For this review, take the finished solid that the model builds, in its own axes (mm). Face numbers are marked on the shaded views. Round coordinates to 2 decimals unless told otherwise and drop trailing zeros. Order: outer loops, then holes, each group sorted by start corner. A loop starts at its lowest first (then second) coordinate and runs counter-clockwise, first axis right, second up. Notation, with made-up numbers: M 67.25,44 L 103.25,44 A34 cw 103.25,81 Z; hole C 32.25,26 d3. An arc over 180 degrees is marked long. Use a Markdown table: item, result.
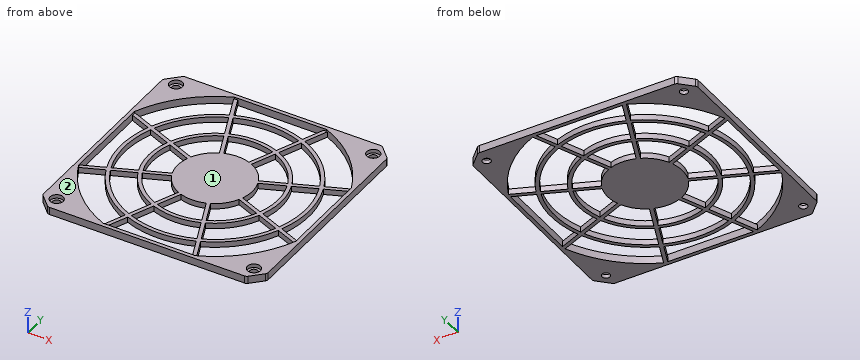
from build123d import *

# Parameters (mm, degrees)
SKETCH1_W           = 120
SKETCH1_H           = 120
SKETCH1_R           = 2.15
BOSS_EXTRUDE1_DEPTH = 4
CHAMFER1_SIZE       = 7
SKETCH2_R           = 20
BOSS_EXTRUDE2_DEPTH = 3
SKETCH3_R           = 50.25
SKETCH3_R_2         = 48.25
SKETCH3_R_3         = 35.5
SKETCH3_R_4         = 33.5
EXTRUDE_THIN1_DEPTH = 3
FILLET1_R           = 2
SKETCH4_R           = 3.5
CUT_EXTRUDE1_DEPTH  = 2


with BuildPart() as part:
    # Sketch1 → Boss-Extrude1 (new body)
    with BuildSketch(Plane.XY):
        Rectangle(SKETCH1_W, SKETCH1_H)
        with Locations((-52.7, 52.7)):
            Circle(SKETCH1_R, mode=Mode.SUBTRACT)
        with Locations((52.7, 52.7)):
            Circle(SKETCH1_R, mode=Mode.SUBTRACT)
        with Locations((-52.7, -52.7)):
            Circle(SKETCH1_R, mode=Mode.SUBTRACT)
        with Locations((52.7, -52.7)):
            Circle(SKETCH1_R, mode=Mode.SUBTRACT)
        with BuildLine():
            Line((-24.596747752, 58), (24.596747752, 58))
            ThreePointArc((24.596747752, 58), (44.547727215, 44.547727215), (58, 24.596747752))
            Line((58, 24.596747752), (58, -24.596747752))
            ThreePointArc((58, -24.596747752), (44.547727215, -44.547727215), (24.596747752, -58))
            Line((24.596747752, -58), (-24.596747752, -58))
            ThreePointArc((-24.596747752, -58), (-44.547727215, -44.547727215), (-58, -24.596747752))
            Line((-58, -24.596747752), (-58, 24.596747752))
            ThreePointArc((-58, 24.596747752), (-44.547727215, 44.547727215), (-24.596747752, 58))
        make_face(mode=Mode.SUBTRACT)
    extrude(amount=BOSS_EXTRUDE1_DEPTH)

    # Chamfer1
    chamfer1_edges = [part.edges().sort_by_distance(p)[0] for p in [
        (60, -60, 2),
        (-60, -60, 2),
        (-60, 60, 2),
        (60, 60, 2),
    ]]
    chamfer(chamfer1_edges, length=CHAMFER1_SIZE)



with BuildPart() as body_2:
    # Sketch2 → Boss-Extrude2 (new body)
    with BuildSketch(Plane.XY):
        Circle(SKETCH2_R)
    extrude(amount=BOSS_EXTRUDE2_DEPTH)


with BuildPart() as part_1:
    add(part.part)

    add(body_2.part)  # Extrude-Thin1 merges body 2
    # Sketch3 → Extrude-Thin1 (add)
    # profile 1 of 10: a face of its own
    with BuildSketch(Plane.XY):
        Circle(SKETCH3_R)
        Circle(SKETCH3_R_2, mode=Mode.SUBTRACT)
    # profile 2 of 10: a face of its own
    with BuildSketch(Plane.XY):
        Circle(SKETCH3_R_3)
        Circle(SKETCH3_R_4, mode=Mode.SUBTRACT)
    # profile 3 of 10: a face of its own
    with BuildSketch(Plane.XY):
        Polygon((7.620839599, 15.785208387), (25.12860663, 58.052696999), (23.280847565, 58.818063864), (5.773080534, 16.550575251), align=None)
    # profile 4 of 10: a face of its own
    with BuildSketch(Plane.XY):
        Polygon((16.550575251, 5.773080534), (58.818063864, 23.280847565), (58.052696999, 25.12860663), (15.785208387, 7.620839599), align=None)
    # profile 5 of 10: a face of its own
    with BuildSketch(Plane.XY):
        Polygon((15.785208387, -7.620839599), (58.052696999, -25.12860663), (58.818063864, -23.280847565), (16.550575251, -5.773080534), align=None)
    # profile 6 of 10: a face of its own
    with BuildSketch(Plane.XY):
        Polygon((5.773080534, -16.550575251), (23.280847565, -58.818063864), (25.12860663, -58.052696999), (7.620839599, -15.785208387), align=None)
    # profile 7 of 10: a face of its own
    with BuildSketch(Plane.XY):
        Polygon((-7.620839599, -15.785208387), (-25.12860663, -58.052696999), (-23.280847565, -58.818063864), (-5.773080534, -16.550575251), align=None)
    # profile 8 of 10: a face of its own
    with BuildSketch(Plane.XY):
        Polygon((-16.550575251, -5.773080534), (-58.818063864, -23.280847565), (-58.052696999, -25.12860663), (-15.785208387, -7.620839599), align=None)
    # profile 9 of 10: a face of its own
    with BuildSketch(Plane.XY):
        Polygon((-15.785208387, 7.620839599), (-58.052696999, 25.12860663), (-58.818063864, 23.280847565), (-16.550575251, 5.773080534), align=None)
    # profile 10 of 10: a face of its own
    with BuildSketch(Plane.XY):
        Polygon((-5.773080534, 16.550575251), (-23.280847565, 58.818063864), (-25.12860663, 58.052696999), (-7.620839599, 15.785208387), align=None)
    extrude(amount=EXTRUDE_THIN1_DEPTH)

    # Fillet1
    fillet1_edges = [part_1.edges().sort_by_distance(p)[0] for p in [
        (60, -53, 2),
        (60, 53, 2),
        (53, 60, 2),
        (-53, 60, 2),
        (-60, -53, 2),
        (-60, 53, 2),
        (-53, -60, 2),
        (53, -60, 2),
    ]]
    fillet(fillet1_edges, radius=FILLET1_R)

    # Sketch4 → Cut-Extrude1 (cut)
    with BuildSketch(Plane.XY.offset(4)):
        with Locations((-52.7, 52.7)):
            Circle(SKETCH4_R)
        with Locations((52.7, 52.7)):
            Circle(SKETCH4_R)
        with Locations((52.7, -52.7)):
            Circle(SKETCH4_R)
        with Locations((-52.7, -52.7)):
            Circle(SKETCH4_R)
    extrude(amount=-CUT_EXTRUDE1_DEPTH, mode=Mode.SUBTRACT)


solid = part_1.part
Q1. Clearance check with flat-ended pins moving along their axes: pin 1 (2 mm diameter, centred on x = -52, y = -54, fed in from +Z); pin 2 (10 mm diameter, centred on x = -15.5, y = -3, fed in from +Z). State where each tip first meets the part, or that it passes through.
Determined:
| item | result |
|---|---|
| pin 1 | stops at z = 2 |
| pin 2 | stops at z = 3 |
Q2. Add section A-A (x = 38). Write out the cut boundary in (y, z).
Determined:
| item | result |
|---|---|
| outline | M -60,0 L -50.25,0 L -50.25,4 L -60,4 Z; M -32.88,0 L -29.73,0 L -29.73,3 L -32.88,3 Z; M -16.82,0 L -14.66,0 L -14.66,3 L -16.82,3 Z; M 14.66,0 L 16.82,0 L 16.82,3 L 14.66,3 Z; M 29.73,0 L 32.88,0 L 32.88,3 L 29.73,3 Z; M 50.25,0 L 60,0 L 60,4 L 50.25,4 Z |
Q3. Add section B-B (y = 29). Give the number of separate pieces and of enclosed holes in the cut face, then the cut area to 3 significant figures.
Determined:
| item | result |
|---|---|
| separate pieces | 8 |
| enclosed holes | 0 |
| area | 82.6 mm^2 |
Q4. Wall thickness on line 1 along X through (y, z) = (50.5, 0.6); line 2 along X through (y, z) = (51, 3.75); line 3 along X through (y, z) = (-52.7, 1.05): over which ranges is each line inside the solid? List them lowest first. Write a range as [from, to].
Determined:
| item | result |
|---|---|
| line 1 | x = [-60, -37.67], [-22, -19.84], [19.84, 22], [37.67, 60] |
| line 2 | x = [-60, -55.76], [-49.64, -36.99], [36.99, 49.64], [55.76, 60] |
| line 3 | x = [-59.93, -54.85], [-50.55, -34.52], [-22.91, -20.75], [20.75, 22.91], [34.52, 50.55], [54.85, 59.93] |
Q5. Draft analysis for pull direction X (two halves, no side actions). For the marked faces 1 and 2, state which applies: pulls with the +X half, pulls with the -X half, needs draft (parallel to the pull), parting line crosses it, or undercut.
Determined:
| item | result |
|---|---|
| face 1 | undercut |
| face 2 | needs draft |
